```python
from build123d import *

# Parameters (mm, degrees)
SKETCH1_W           = 150
SKETCH1_H           = 76
BOSS_EXTRUDE1_DEPTH = 10
SKETCH2_W           = 126
SKETCH2_H           = 68
CUT_EXTRUDE1_DEPTH  = 0.2
FILLET1_R           = 8


with BuildPart() as part:
    # Sketch1 → Boss-Extrude1 (new body)
    with BuildSketch(Plane(origin=(0, 0, 0), x_dir=(1, 0, 0), z_dir=(0, 1, 0))):
        with Locations((75, 38)):
            Rectangle(SKETCH1_W, SKETCH1_H)
    extrude(amount=BOSS_EXTRUDE1_DEPTH)

    # Sketch2 → Cut-Extrude1 (cut)
    with BuildSketch(Plane(origin=(0, 10, 0), x_dir=(1, 0, 0), z_dir=(0, 1, 0))):
        with Locations((71, 38)):
            Rectangle(SKETCH2_W, SKETCH2_H)
        with BuildLine():
            Line((138, 21), (138, 55))
            ThreePointArc((138, 55), (142, 59), (146, 55))
            Line((146, 55), (146, 21))
            ThreePointArc((146, 21), (142, 17), (138, 21))
        make_face()
        with BuildLine():
            Line((5, 55), (5, 21))
            ThreePointArc((5, 21), (3.5, 19.5), (2, 21))
            Line((2, 21), (2, 55))
            ThreePointArc((2, 55), (3.5, 56.5), (5, 55))
        make_face()
    extrude(amount=-CUT_EXTRUDE1_DEPTH, mode=Mode.SUBTRACT)

    # Fillet1
    fillet1_edges = [part.edges().sort_by_distance(p)[0] for p in [
        (0, 5, -76),
        (150, 5, -76),
        (150, 5, 0),
        (0, 5, 0),
    ]]
    fillet(fillet1_edges, radius=FILLET1_R)


solid = part.part
```
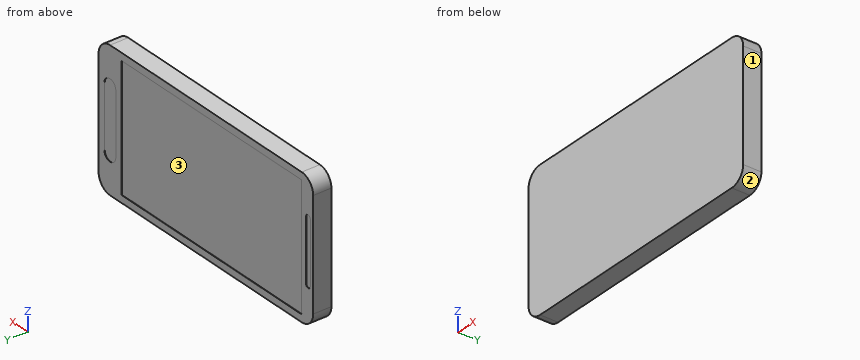
The model under review builds one solid part; all positions refer to its coordinate system, in mm. Face numbers are marked on the shaded views. Give positions to 0.01 mm unless a question says otherwise; leave off trailing zeros. Loops run counter-clockwise (first coordinate to the right, second up) from the corner with the lowest first, then second, coordinate; pieces in that order, holes last. Notation, with made-up numbers: (41, 8) -> (58, 8) arc R5 ccw to (58, 14) -> close; hole circle Ø4 at (2.5, 74). An arc over 180 degrees is marked (long way). Use CSV: the item, a comma, the result in double quotes.
1. For P1, Ø4, axis at x = 143.5, z = -46.5, coming from the +Y side; P2, Ø3.5, axis at x = 3.5, z = -38.5, coming from the +Y side, all flat-tipped, find the tip position at first contact; note any pin that passes through.
Result:
P1,"stops at y = 9.8"
P2,"stops at y = 10"
2. The part is to be moulded in two halves that separate along Z. For the marked faces 1, 2 and 3, say which applies: +Z half, -Z half, draft (parallel to the pull), parting line (faces both ways), or undercut.
Result:
face 1,"draft"
face 2,"-Z half"
face 3,"undercut"
3. Consider section A-A, the plane x = 35. Write out the cut boundary in (y, z), then the cut area to 3 significant figures.
Result:
outline,"(0, -76) -> (10, -76) -> (10, -72) -> (9.8, -72) -> (9.8, -4) -> (10, -4) -> (10, 0) -> (0, 0) -> close"
area,"746 mm²"
4. To check wall thickness, follow probe 1 along Y at (x, z) = (70.5, -27); probe 2 along X at (y, z) = (6.25, -69.5). State the ranges of each line that lie inside material, in increasing order. Write a range as from..to.
Result:
probe 1,"y = 0..9.8"
probe 2,"x = 0.14..149.86"
5. Consider section B-B, the plane z = -28. Write out the cut boundary in (x, y).
Result:
outline,"(0, 0) -> (150, 0) -> (150, 10) -> (146, 10) -> (146, 9.8) -> (138, 9.8) -> (138, 10) -> (134, 10) -> (134, 9.8) -> (8, 9.8) -> (8, 10) -> (5, 10) -> (5, 9.8) -> (2, 9.8) -> (2, 10) -> (0, 10) -> close"
6. Consider section C-C, the plane x = 3.5. Write out the cut boundary in (y, z), then the cut area to 3 significant figures.
Result:
outline,"(0, -74.61) -> (10, -74.61) -> (10, -56.5) -> (9.8, -56.5) -> (9.8, -19.5) -> (10, -19.5) -> (10, -1.39) -> (0, -1.39) -> close"
area,"725 mm²"
